Part model, mm, in its own coordinate system. A direction names the side the tool comes from. Coordinates: 2 decimals unless noted, no trailing zeros. Order: outer loops, then holes, each group sorted by start corner. A loop starts at its lowest first (then second) coordinate and runs counter-clockwise, first axis right, second up. Notation, with made-up numbers: M 13.5,-40 L 40.5,-40 A23 cw 40.5,-32 Z; hole C -33,73 d11. An arc over 180 degrees is marked long. Answer in a Markdown table with one row per item. Add a question column.
from build123d import *

# Parameters (mm, degrees)
BOSS_EXTRUDE2_DEPTH = 6.35
SKETCH2_R           = 3.175
CUT_EXTRUDE1_DEPTH  = 7.35
SKETCH7_R           = 2.286
CUT_EXTRUDE3_DEPTH  = 12.7
SKETCH8_R           = 2.286
CUT_EXTRUDE4_DEPTH  = 7.35
SKETCH9_W           = 129.404437756
SKETCH9_H           = 7.62
CUT_EXTRUDE5_DEPTH  = 7.35
SKETCH10_R          = 4.826
SKETCH10_R_2        = 2.286
BOSS_EXTRUDE3_DEPTH = 3.81
CUT_EXTRUDE6_DEPTH  = 3.175


with BuildPart() as part:
    # Sketch1 → Boss-Extrude2 (new body)
    with BuildSketch(Plane(origin=(0, 0, 0), x_dir=(1, 0, 0), z_dir=(0, 1, 0))):
        with BuildLine():
            Line((0, 0), (0, 25.4))
            ThreePointArc((0, 25.4), (3.719743879, 34.380256121), (12.7, 38.1))
            Line((12.7, 38.1), (190.5, 38.1))
            ThreePointArc((190.5, 38.1), (199.480256121, 34.380256121), (203.2, 25.4))
            Line((203.2, 25.4), (203.2, -152.4))
            ThreePointArc((203.2, -152.4), (199.480256121, -161.380256121), (190.5, -165.1))
            Line((190.5, -165.1), (12.7, -165.1))
            ThreePointArc((12.7, -165.1), (3.719743879, -161.380256121), (0, -152.4))
            Line((0, -152.4), (0, -127))
            Line((0, -127), (181.61, -127))
            Line((181.61, -127), (181.61, 0))
            Line((181.61, 0), (0, 0))
        make_face()
    extrude(amount=BOSS_EXTRUDE2_DEPTH)

    # Sketch2 → Cut-Extrude1 (cut, through all)
    with BuildSketch(Plane(origin=(0, 6.35, 0), x_dir=(1, 0, 0), z_dir=(0, 1, 0))):
        with Locations((12.7, 25.4)):
            Circle(SKETCH2_R)
        with Locations((190.5, 25.4)):
            Circle(SKETCH2_R)
        with Locations((190.5, -152.4)):
            Circle(SKETCH2_R)
        with Locations((12.7, -152.4)):
            Circle(SKETCH2_R)
    extrude(amount=-CUT_EXTRUDE1_DEPTH, mode=Mode.SUBTRACT)

    # Sketch7 → Cut-Extrude3 (cut)
    with BuildSketch(Plane(origin=(0, 6.35, 0), x_dir=(1, 0, 0), z_dir=(0, 1, 0))):
        with Locations((192.024, -101.092)):
            Circle(SKETCH7_R)
        with Locations((192.024, -91.186)):
            Circle(SKETCH7_R)
        with Locations((192.024, -35.814)):
            Circle(SKETCH7_R)
        with Locations((192.024, -25.908)):
            Circle(SKETCH7_R)
    extrude(amount=-CUT_EXTRUDE3_DEPTH, mode=Mode.SUBTRACT)

    # Sketch8 → Cut-Extrude4 (cut, through all)
    with BuildSketch(Plane(origin=(0, 0, 0), x_dir=(-1, 0, 0), z_dir=(0, -1, 0))):
        with Locations((-24.197781122, 13.902218878)):
            Circle(SKETCH8_R)
        with Locations((-24.197781122, -140.902218878)):
            Circle(SKETCH8_R)
        with Locations((-179.002218878, -140.902218878)):
            Circle(SKETCH8_R)
        with Locations((-179.002218878, 13.902218878)):
            Circle(SKETCH8_R)
    extrude(amount=-CUT_EXTRUDE4_DEPTH, mode=Mode.SUBTRACT)

    # Sketch9 → Cut-Extrude5 (cut, through all)
    with BuildSketch(Plane(origin=(0, 6.35, 0), x_dir=(1, 0, 0), z_dir=(0, 1, 0))):
        with Locations((101.6, 3.81)):
            Rectangle(SKETCH9_W, SKETCH9_H)
        with Locations((101.6, -130.81)):
            Rectangle(SKETCH9_W, SKETCH9_H)
    extrude(amount=-CUT_EXTRUDE5_DEPTH, mode=Mode.SUBTRACT)

    # Sketch10 → Boss-Extrude3 (add)
    with BuildSketch(Plane(origin=(0, 0, 0), x_dir=(-1, 0, 0), z_dir=(0, -1, 0))):
        with Locations((-44.45, 12.7)):
            Circle(SKETCH10_R)
        with Locations((-44.45, 12.7)):
            Circle(SKETCH10_R_2, mode=Mode.SUBTRACT)
        with Locations((-158.75, 12.7)):
            Circle(SKETCH10_R)
        with Locations((-158.75, 12.7)):
            Circle(SKETCH10_R_2, mode=Mode.SUBTRACT)
        with Locations((-158.75, -139.7)):
            Circle(SKETCH10_R)
        with Locations((-158.75, -139.7)):
            Circle(SKETCH10_R_2, mode=Mode.SUBTRACT)
        with Locations((-44.45, -139.7)):
            Circle(SKETCH10_R)
        with Locations((-44.45, -139.7)):
            Circle(SKETCH10_R_2, mode=Mode.SUBTRACT)
    extrude(amount=BOSS_EXTRUDE3_DEPTH)

    # Sketch11 → Cut-Extrude6 (cut)
    with BuildSketch(Plane(origin=(0, 6.35, 0), x_dir=(1, 0, 0), z_dir=(0, 1, 0))):
        Polygon((0, 0), (36.897781122, 0), (36.897781122, 7.62), (166.302218878, 7.62), (166.302218878, 0), (181.61, 0), (181.61, 6.35), (172.652218878, 6.35), (172.652218878, 13.97), (30.547781122, 13.97), (30.547781122, 6.35), (0, 6.35), align=None)
        Polygon((0, -133.35), (0, -127), (36.897781122, -127), (36.897781122, -134.62), (166.302218878, -134.62), (166.302218878, -127), (181.61, -127), (181.61, -133.35), (172.652218878, -133.35), (172.652218878, -140.97), (30.547781122, -140.97), (30.547781122, -133.35), align=None)
    extrude(amount=-CUT_EXTRUDE6_DEPTH, mode=Mode.SUBTRACT)


solid = part.part
(1) Slice it at C-C (y = 4.75). State how many separate pieces and enclosed holes the cut face has, and give its area (3 significant figures).
(2) Pull direction Z, two halves, no side cores. Call faces 3 (the flat face through (203.2, 3, 62)), 4 (the cylindrical face through (199.58, 3.13, 161.28)), 5 (the flat face through (159, 0, 140)): pulls with the +Z half, pulls with the -Z half, needs draft (parallel to the pull), parting line crosses it, or undercut.
(3) Drop flat-ended pins along their axis: P1, Ø3, axis at x = 89, z = 144, coming from the -Y side; P2, Ø3.5, axis at x = 10.5, y = 4, coming from the -Z side; P3, Ø3, axis at y = -2.5, z = 144, coming from the +X side. Give the stop position or say it passes through.
(4) Wall check: line 1 (X direction, y = 0.5, z = -13.5); line 2 (X direction, y = 5, z = 35.5); line 3 (Z direction, x = 153, y = 2). Give the ranges that are in metal, low to high.
(5) Slice it at A-A (x = 143). List the corners of the cut face in (y, z) (3 decimals).
(6) Slice it at B-B (z = 68). List the corners of the cut face in (x, y), and give its area (3 significant figures).
(7) 3-axis set-ups, long thin cutter, end or side, ignore diameter. For faces 1 (the flat face through (100, 3, -38.1)), 2 (the flat face through (44, 0, 140)): which of +Z, -Z, +X, -X, +Y, -Y reach the whole face in a straight line?
Computed:
| question | item | result |
|---|---|---|
| 1 | separate pieces | 1 |
| 1 | enclosed holes | 12 |
| 1 | area | 13,400 mm^2 |
| 2 | face 3 | needs draft |
| 2 | face 4 | pulls with the +Z half |
| 2 | face 5 | undercut |
| 3 | P1 | stops at y = 0 |
| 3 | P2 | stops at z = -38.09 |
| 3 | P3 | stops at x = 162.68 |
| 4 | line 1 | x = 0 to 21.95, 26.45 to 176.75, 181.25 to 203.2 |
| 4 | line 2 | x = 181.61 to 189.76, 194.29 to 203.2 |
| 4 | line 3 | z = -38.1 to -7.62, 134.62 to 165.1 |
| 5 | outline | M 0,-38.1 L 6.35,-38.1 L 6.35,-13.97 L 3.175,-13.97 L 3.175,-7.62 L 0,-7.62 Z; M 0,134.62 L 3.175,134.62 L 3.175,140.97 L 6.35,140.97 L 6.35,165.1 L 0,165.1 Z |
| 6 | outline | M 181.61,0 L 203.2,0 L 203.2,6.35 L 181.61,6.35 Z |
| 6 | area | 137 mm^2 |
| 7 | face 1 | -Z, +X, -X, +Y, -Y |
| 7 | face 2 | -Y |
